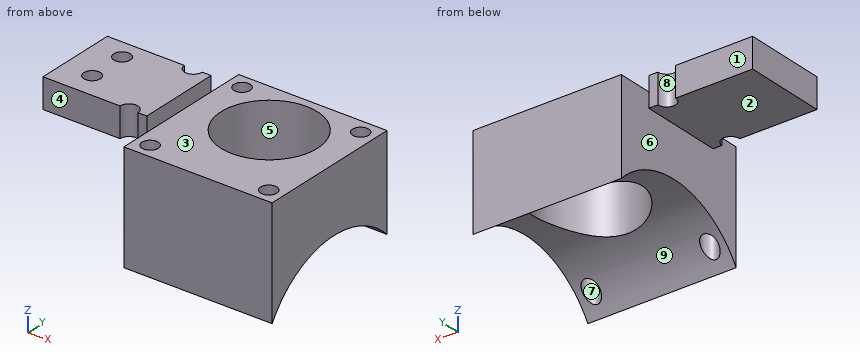
```python
from build123d import *
from build123d.topology import SkipClean

# Parameters (mm, degrees)
SKETCH1_W               = 50
SKETCH1_H               = 50
SKETCH1_R               = 2.75
SKETCH1_R_2             = 16.3
BOSS_EXTRUDE1_DEPTH     = 53.6
CUT_EXTRUDE1_DEPTH      = 66.015075175
CUT_EXTRUDE1_DEPTH_BACK = 66.015075175
SKETCH2_R               = 31.75
BOSS_EXTRUDE3_START     = 35
BOSS_EXTRUDE3_DEPTH     = 35
SKETCH9_R               = 3
CUT_EXTRUDE5_DEPTH      = 85.864362462
CUT_EXTRUDE6_DEPTH      = 76.433606288
CUT_EXTRUDE6_DEPTH_BACK = 10
SKETCH10_R              = 2.8
CUT_EXTRUDE8_START      = -5
SKETCH13_R              = 2.8
CUT_EXTRUDE8_DEPTH      = 71.433606288
BOSS_EXTRUDE4_START     = 5
SKETCH13_3_R            = 2.8
BOSS_EXTRUDE4_DEPTH     = 5
CUT_EXTRUDE9_DEPTH      = 5
CUT_EXTRUDE9_DEPTH_BACK = 5
SKETCH13_4_R            = 2.8


with BuildPart() as part:
    # Sketch1 → Boss-Extrude1 (new body)
    with BuildSketch(Plane.XY):
        with Locations((0, -2)):
            Rectangle(SKETCH1_W, SKETCH1_H)
        with Locations((-20, 18)):
            Circle(SKETCH1_R, mode=Mode.SUBTRACT)
        with Locations((20, 18)):
            Circle(SKETCH1_R, mode=Mode.SUBTRACT)
        with Locations((20, -22)):
            Circle(SKETCH1_R, mode=Mode.SUBTRACT)
        with Locations((-20, -22)):
            Circle(SKETCH1_R, mode=Mode.SUBTRACT)
        with Locations((0, 4)):
            Circle(SKETCH1_R_2, mode=Mode.SUBTRACT)
    extrude(amount=BOSS_EXTRUDE1_DEPTH)

    # Sketch2 → Cut-Extrude1 (cut, two sides: drawn at the far end of the back side and taken through both)
    with BuildSketch(Plane(origin=(0, 0, 0), x_dir=(0, 0, -1), z_dir=(1, 0, 0)).offset(-CUT_EXTRUDE1_DEPTH_BACK)):
        Circle(SKETCH2_R)
    extrude(amount=CUT_EXTRUDE1_DEPTH + CUT_EXTRUDE1_DEPTH_BACK, mode=Mode.SUBTRACT)

    # Sketch4 → Boss-Extrude3 (add)
    with SkipClean():  # the faces are left unmerged after this step: merging them gives an invalid solid
        with BuildSketch(Plane(origin=(25, 0, 0), x_dir=(0, 0, -1), z_dir=(1, 0, 0)).offset(BOSS_EXTRUDE3_START)):
            with BuildLine():
                Line((-53.6, 11), (-53.6, -17))
                Line((-53.6, -17), (-26.815340759, -17))
                ThreePointArc((-26.815340759, -17), (-31.573087709, -3.347033393), (-29.783594477, 11))
                Line((-29.783594477, 11), (-53.6, 11))
            make_face()
        boss_extrude3 = extrude(amount=-BOSS_EXTRUDE3_DEPTH)

    # Sketch9 → Cut-Extrude5 (cut, symmetric)
    with SkipClean():  # the faces are left unmerged after this step: merging them gives an invalid solid
        with BuildSketch(Plane.XY):
            with Locations((31, 11)):
                Circle(SKETCH9_R)
            with Locations((31, -17)):
                Circle(SKETCH9_R)
        cut_extrude5 = extrude(amount=CUT_EXTRUDE5_DEPTH, both=True, mode=Mode.SUBTRACT)

    # Sketch10 → Cut-Extrude6 (cut, two sides: drawn at the far end of the back side and taken through both)
    with SkipClean():  # the faces are left unmerged after this step: merging them gives an invalid solid
        with BuildSketch(Plane.XY.offset(53.6).offset(-CUT_EXTRUDE6_DEPTH_BACK)):
            with Locations(Location((50, 4.5, 0), (0, 0, 180))):
                Circle(SKETCH10_R)
            with Locations(Location((50, -8.5, 0), (0, 0, 180))):
                Circle(SKETCH10_R)
        extrude(amount=CUT_EXTRUDE6_DEPTH + CUT_EXTRUDE6_DEPTH_BACK, mode=Mode.SUBTRACT)

    # Sketch13 → Cut-Extrude8 (cut, through all)
    # profile 1 of 3: a face of its own
    with BuildSketch(Plane.XY.offset(53.6).offset(CUT_EXTRUDE8_START)):
        with BuildLine():
            Line((25, 11), (25, -17))
            Line((25, -17), (28, -17))
            ThreePointArc((28, -17), (31, -14), (34, -17))
            Line((34, -17), (60, -17))
            Line((60, -17), (60, 11))
            Line((60, 11), (34, 11))
            ThreePointArc((34, 11), (31, 8), (28, 11))
            Line((28, 11), (25, 11))
        make_face()
        with Locations(Location((50, 4.5, 0), (0, 0, 180))):
            Circle(SKETCH13_R, mode=Mode.SUBTRACT)
        with Locations(Location((50, -8.5, 0), (0, 0, 180))):
            Circle(SKETCH13_R, mode=Mode.SUBTRACT)
    # profile 2 of 3: a face of its own
    with BuildSketch(Plane.XY.offset(53.6).offset(CUT_EXTRUDE8_START)):
        with Locations(Location((50, -8.5, 0), (0, 0, 180))):
            Circle(SKETCH13_R)
    # profile 3 of 3: a face of its own
    with BuildSketch(Plane.XY.offset(53.6).offset(CUT_EXTRUDE8_START)):
        with Locations(Location((50, 4.5, 0), (0, 0, 180))):
            Circle(SKETCH13_R)
    cut_extrude8 = extrude(amount=-CUT_EXTRUDE8_DEPTH, mode=Mode.SUBTRACT)

    # Sketch13_3 → Boss-Extrude4 (add)
    with SkipClean():  # the faces are left unmerged after this step: merging them gives an invalid solid
        with BuildSketch(Plane.XY.offset(53.6).offset(BOSS_EXTRUDE4_START)):
            with BuildLine():
                Line((60, 11), (60, -17))
                Line((60, -17), (34, -17))
                ThreePointArc((34, -17), (31, -14), (28, -17))
                Line((28, -17), (25, -17))
                Line((25, -17), (25, 11))
                Line((25, 11), (28, 11))
                ThreePointArc((28, 11), (31, 8), (34, 11))
                Line((34, 11), (60, 11))
            make_face()
            with Locations(Location((50, 4.5, 0), (0, 0, 180))):
                Circle(SKETCH13_3_R, mode=Mode.SUBTRACT)
            with Locations(Location((50, -8.5, 0), (0, 0, 180))):
                Circle(SKETCH13_3_R, mode=Mode.SUBTRACT)
        boss_extrude4 = extrude(amount=-BOSS_EXTRUDE4_DEPTH)
    add(part.part.scale(1), mode=Mode.REPLACE)  # the faces are merged on a copy

    # Mirror3: Boss-Extrude3, Cut-Extrude5, Cut-Extrude8, Boss-Extrude4 across plane
    with SkipClean():  # the faces are left unmerged after this step: merging them gives an invalid solid
        add(boss_extrude3.mirror(Plane(origin=(0, 0, 0), x_dir=(0, 0, 1), z_dir=(1, 0, 0))))
        add(cut_extrude5.mirror(Plane(origin=(0, 0, 0), x_dir=(0, 0, 1), z_dir=(1, 0, 0))), mode=Mode.SUBTRACT)
        add(cut_extrude8.mirror(Plane(origin=(0, 0, 0), x_dir=(0, 0, 1), z_dir=(1, 0, 0))), mode=Mode.SUBTRACT)
        add(boss_extrude4.mirror(Plane(origin=(0, 0, 0), x_dir=(0, 0, 1), z_dir=(1, 0, 0))))
    add(part.part.scale(1), mode=Mode.REPLACE)  # the faces are merged on a copy

    # Sketch13_4 → Cut-Extrude9 (cut, two sides: drawn at the far end of the back side and taken through both)
    with SkipClean():  # the faces are left unmerged after this step: merging them gives an invalid solid
        with BuildSketch(Plane.XY.offset(53.6).offset(-CUT_EXTRUDE9_DEPTH_BACK)):
            with BuildLine():
                Line((60, 11), (60, -17))
                Line((60, -17), (34, -17))
                ThreePointArc((34, -17), (31, -14), (28, -17))
                Line((28, -17), (25, -17))
                Line((25, -17), (25, 11))
                Line((25, 11), (28, 11))
                ThreePointArc((28, 11), (31, 8), (34, 11))
                Line((34, 11), (60, 11))
            make_face()
            with Locations((50, 4.5)):
                Circle(SKETCH13_4_R, mode=Mode.SUBTRACT)
            with Locations((50, -8.5)):
                Circle(SKETCH13_4_R, mode=Mode.SUBTRACT)
        extrude(amount=CUT_EXTRUDE9_DEPTH + CUT_EXTRUDE9_DEPTH_BACK, mode=Mode.SUBTRACT)


solid = part.part
```
Design review of the part built by this model. Coordinates are the model's own, in mm. Face numbers are marked on the shaded views. A direction names the side the tool comes from. Round coordinates to 2 decimals unless told otherwise and drop trailing zeros. Order: outer loops, then holes, each group sorted by start corner. A loop starts at its lowest first (then second) coordinate and runs counter-clockwise, first axis right, second up. Notation, with made-up numbers: (67, 17) - (87, 17) arc R16 ccw to (87, 47) - close; hole circle Ø1 at (-14.5, 34). An arc over 180 degrees is marked (long way). Return JSON: item names as keys, results as strings.
Q1. Consider section D-D on x = -50. Write out the cut boundary in (y, z), plus the area to 3 significant figures.
Computed values:
{"outline": "(-17, 48.6) - (11, 48.6) - (11, 58.6) - (7.3, 58.6) - (7.3, 53.6) - (1.7, 53.6) - (1.7, 58.6) - (-5.7, 58.6) - (-5.7, 53.6) - (-11.3, 53.6) - (-11.3, 58.6) - (-17, 58.6) - close", "area": "224 mm2"}
Q2. Consider section B-B on x = -6.5. Write out the cut boundary in (y, z), plus the area to 3 significant figures.
Computed values:
{"outline": "(-27, 16.71) arc R31.75 cw to (-10.95, 29.8) - (-10.95, 53.6) - (-27, 53.6) - close; (18.95, 25.48) arc R31.75 cw to (23, 21.89) - (23, 53.6) - (18.95, 53.6) - close", "area": "584 mm2"}
Q3. Consider section A-A on z = 39. Write out the cut boundary in (x, y).
Computed values:
{"outline": "(-25, -27) - (25, -27) - (25, 23) - (-25, 23) - close; hole circle Ø5.5 at (-20, -22); hole circle Ø5.5 at (-20, 18); hole circle Ø32.6 at (0, 4); hole circle Ø5.5 at (20, -22); hole circle Ø5.5 at (20, 18)"}
Q4. Machinability: for the marked faces 1, 2, 3, 4 and 5, which of the approach directions +Z, -Z, +X, -X, +Y, -Y give a long, thin tool a straight path to every point of the face, cutting with its end or side? Answer none if there is none.
Computed values:
{"face 1": "+Z, -Z, -X, +Y", "face 2": "-Z, -X, +Y, -Y", "face 3": "+Z, +X, +Y, -Y", "face 4": "+Z, -Z, -X, -Y", "face 5": "+Z, -Z"}
Q5. Wall thickness on L1, parallel to X at y = -22, z = 27; L2, parallel to Y at x = -50, z = 55.9; L3, parallel to Y at x = 20, z = 38: over which ranges is each line inside the solid? List them lowest first. Write a range as [from, to].
Computed values:
{"L1": "x = [-25, -22.75], [-17.25, 17.25], [22.75, 25]", "L2": "y = [-17, -11.3], [-5.7, 1.7], [7.3, 11]", "L3": "y = [-27, -24.75], [-19.25, 15.25], [20.75, 23]"}
Q6. For pin 1 Ø1.5 at (x, y) = (-7.5, 15.5) entering from +Z; pin 2 Ø8.5 at (x, y) = (-40.5, -4) entering from -Z; pin 3 Ø11 at (x, z) = (-42.5, 54) entering from +Y; pin 4 Ø25 at (x, y) = (-2, -5.5) entering from +Z, all flat-tipped, find the tip position at first contact; note any pin that passes through.
Computed values:
{"pin 1": "passes through", "pin 2": "stops at z = 48.6", "pin 3": "stops at y = 11", "pin 4": "stops at z = 53.6"}
Q7. Consider section C-C on y = -22. Write out the cut boundary in (x, z), plus the area to 3 significant figures.
Computed values:
{"outline": "(-25, 22.89) - (-22.75, 22.89) - (-22.75, 53.6) - (-25, 53.6) - close; (-17.25, 22.89) - (17.25, 22.89) - (17.25, 53.6) - (-17.25, 53.6) - close; (22.75, 22.89) - (25, 22.89) - (25, 53.6) - (22.75, 53.6) - close", "area": "1,200 mm2"}
Q8. The part is to be moulded in two halves that separate along Y. For the marked faces 6, 7, 8 and 9, say which applies: pulls with the +Y half, pulls with the -Y half, needs draft (parallel to the pull), parting line crosses it, or undercut.
Computed values:
{"face 6": "needs draft", "face 7": "undercut", "face 8": "pulls with the +Y half", "face 9": "undercut"}
